The model under review builds one solid part; all positions refer to its coordinate system, in mm. A direction names the side the tool comes from. Round coordinates to 2 decimals unless told otherwise and drop trailing zeros. Write each loop counter-clockwise with the first axis right and the second up, starting at its lowest first coordinate (ties: lowest second). Pieces come first, ordered by that corner, then holes. Notation, with made-up numbers: (71, 21.5) - (112, 21.5) arc R36 cw to (112, 57.5) - close; hole circle Ø1 at (66, 47.25). An arc over 180 degrees is marked (long way). One line per question, with ' | ' between items. Start each with the question number.
Autodesk Fusion 360 part; units mm, degrees
sketch "スケッチ1" plane through (0, 0, 0) normal (0, 1, 0) x (1, 0, 0)
  line L0 (115.8209, 0) -> (-126.022, 0) construction
  line L1 (0, -92.6498) -> (0, 100.0832) construction
  circle A0 centre (0, 0) radius 24.5
  circle A1 centre (0, 0) radius 29.5
  circle A2 centre (0, 0) radius 21.5
  line L2 (21.3542, -2.5) -> (-21.3542, -2.5)
  line L3 (21.3542, 2.5) -> (-21.3542, 2.5)
  line L4 (2.5, -21.3542) -> (2.5, 21.3542)
  line L5 (-2.5, 21.4531) -> (-2.5, -21.3542)
  circle A3 centre (0, 0) radius 12.5
  circle A4 centre (0, 0) radius 15.5
  dimension "d1" = 49
  dimension "d2" = 59
  dimension "d3" = 43
  dimension "d4" = 2.5
  dimension "d5" = 2.5
  dimension "d6" = 2.5
  dimension "d7" = 2.5
  dimension "d8" = 25
  dimension "d9" = 31
extrude "押し出し1" add sketch "スケッチ1" along normal blind 2 contours A2 L2 L3 A4 | A2 L4 L5 A4 | L2 L3 A3 A4 | L3 L4 A3 A4 | A2 L4 L5 A4 | L2 L4 A3 A4 | L4 L5 A3 A4 | L2 L3 L4 A3 | L4 L5 A3 A4 | A2 L2 L3 A4 | L3 L5 A3 A4 | L3 L4 L5 A3 | L2 L3 L4 L5 | L2 L5 A3 A4 | L2 L4 L5 A3 | L2 L3 A3 A4 | L2 L3 L5 A3
extrude "押し出し2" add sketch "スケッチ1" along normal blind 30 contours A0
extrude "押し出し3" add sketch "スケッチ1" against normal blind 1.5 from surface at 30 contours A1
1. Machinability: for faces 1 (the face through (-7, 28.5, -24)), 2 (the face through (-2.5, 1, 7)), which of the approach directions +Z, -Z, +X, -X, +Y, -Y give a long, thin tool a straight path to every point of the face, cutting with its end or side? Answer none if there is none.
2. Add section B-B, the plane z = 0. Write out the cut boundary in (x, y).
3. Add section A-A, the plane x = -17. Write out the cut boundary in (y, z).
4. Add section D-D, the plane z = 14. Write out the cut boundary in (x, y).
5. Wall thickness on line 1 along X through (y, z) = (18.5, 0); line 2 along Y through (x, z) = (-13.5, 3.5): over which ranges is each line inside the solid? List them lowest first. Write a range as [from, to].
6. Clearance check with flat-ended pins moving along their axes: P1, Ø1, axis at x = 19.5, y = 0.5, coming from the +Z side; P2, Ø8, axis at x = 6.5, z = 10.5, coming from the +Y side; P3, Ø1, axis at x = 8.5, y = 1.5, coming from the -Z side; P4, Ø3, axis at x = 7, z = 2, coming from the -Y side. State where each tip first meets the part, or that it passes through.
7. The part is to be moulded in two halves that separate along Z. For faces 3 (the face through (2, 30, 22)), 4 (the face through (28.14, 29.26, -8.86)), 5 (the face through (2.5, 1, -7)), say which applies: pulls with the +Z half, pulls with the -Z half, needs draft (parallel to the pull), parting line crosses it, or undercut.
8. Add section C-C, the plane x = 0. Write out the cut boundary in (y, z).
Geometry check:
1) face 1: -Y | face 2: +Y, -Y
2) outline: (-29.5, 28.5) - (-24.5, 28.5) - (-24.5, 0) - (24.5, 0) - (24.5, 28.5) - (29.5, 28.5) - (29.5, 30) - (21.5, 30) - (21.5, 2) - (-21.5, 2) - (-21.5, 30) - (-29.5, 30) - close
3) outline: (0, -17.64) - (28.5, -17.64) - (28.5, -24.11) - (30, -24.11) - (30, -13.16) - (0, -13.16) - close; (0, -2.5) - (2, -2.5) - (2, 2.5) - (0, 2.5) - close; (0, 13.16) - (30, 13.16) - (30, 24.11) - (28.5, 24.11) - (28.5, 17.64) - (0, 17.64) - close
4) outline: (-25.97, 28.5) - (-20.11, 28.5) - (-20.11, 0) - (-16.32, 0) - (-16.32, 30) - (-25.97, 30) - close; (-6.65, 0) - (6.65, 0) - (6.65, 2) - (-6.65, 2) - close; (16.32, 0) - (20.11, 0) - (20.11, 28.5) - (25.97, 28.5) - (25.97, 30) - (16.32, 30) - close
5) line 1: x = [-24.5, -21.5], [21.5, 24.5] | line 2: y = [0, 2]
6) P1: stops at z = 15.47 | P2: stops at y = 2 | P3: stops at z = -23.16 | P4: stops at y = 0
7) face 3: needs draft | face 4: parting line crosses it | face 5: undercut
8) outline: (0, -24.5) - (28.5, -24.5) - (28.5, -29.5) - (30, -29.5) - (30, -21.5) - (2, -21.5) - (2, 21.5) - (30, 21.5) - (30, 29.5) - (28.5, 29.5) - (28.5, 24.5) - (0, 24.5) - close
